Autodesk Inventor part; units mm, degrees
ref_plane "YZ Plane" through (0, 0, 0) normal (1, 0, 0) x (0, 1, 0)
ref_plane "XZ Plane" through (0, 0, 0) normal (0, 1, 0) x (-1, 0, 0)
ref_plane "XY Plane" through (0, 0, 0) normal (0, 0, 1) x (1, 0, 0)
sketch "Sketch1" plane through (0, 0, 0) normal (1, 0, 0) x (0, 1, 0)
  circle A0 centre (0, 0) radius 2.5
extrude "Extrusion1" add sketch "Sketch1" along normal mid plane 3
sketch "Sketch2" plane through (1.5, 0, 0) normal (1, 0, 0) x (0, 0, -1)
  circle A0 centre (0, 0) radius 1.5
extrude "Extrusion2" add sketch "Sketch2" along normal blind 18
fillet "Fillet1" radius 1.2 1 edges at (-1.5, -2.5, 0)
sketch "Sketch3" plane through (0, 0, 0) normal (0, 1, 0) x (-1, 0, 0)
  line L0 (1.5, 1.3) -> (1.5, -1.3)
  line L1 (0.3, -2.5) -> (0.3, 2.5)
  line L2 (1.5, 0.5) -> (0.3, 0.5)
  line L3 (1.5, -0.5) -> (0.3, -0.5)
  line L4 (1.5, -0.5) -> (1.5, 0.5)
  line L5 (0.3, 0.5) -> (0.3, -0.5)
  point P0 (0, 0)
extrude "Extrusion3" cut sketch "Sketch3" along normal mid plane 18
thread "Thread1"
thread "Thread2"
properties part number "parafuso do captador( necessita de reparo)"
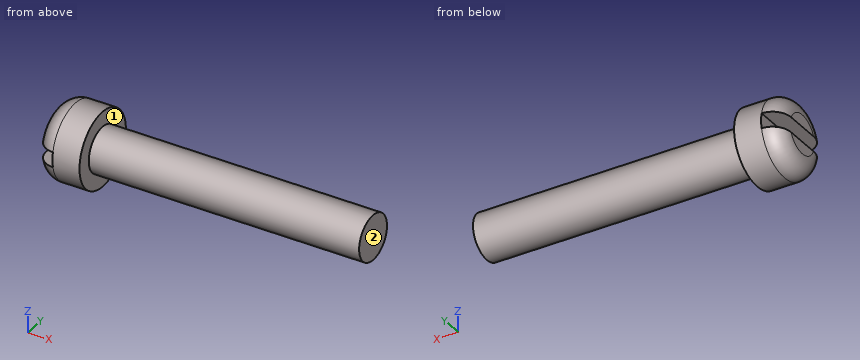
Work out the finished part from the listing and answer in its coordinate system (mm). Face numbers are marked on the shaded views. A direction names the side the tool comes from. Round coordinates to 2 decimals unless told otherwise and drop trailing zeros. Loops run counter-clockwise (first coordinate to the right, second up) from the corner with the lowest first, then second, coordinate; pieces in that order, holes last. Notation, with made-up numbers: M -20,-23.75 L 26,-23.75 A8 cw 26,-14.75 Z; hole C 44.5,68 d5. An arc over 180 degrees is marked long. One line per question, with ' | ' between items.
Q1. Find section B-B, the plane y = 0. Give the vertices of the cut face in (x, z).
Conclusion:
outline: M -1.5,-1.3 A1.2 ccw -0.3,-2.5 L 1.5,-2.5 L 1.5,-1.5 L 19.5,-1.5 L 19.5,1.5 L 1.5,1.5 L 1.5,2.5 L -0.3,2.5 A1.2 ccw -1.5,1.3 L -1.5,0.5 L -0.3,0.5 L -0.3,-0.5 L -1.5,-0.5 Z
Q2. Find section A-A, the plane z = 0. Give the vertices of the cut face in (x, y).
Conclusion:
outline: M -0.3,-2.5 L 1.5,-2.5 L 1.5,-1.5 L 19.5,-1.5 L 19.5,1.5 L 1.5,1.5 L 1.5,2.5 L -0.3,2.5 Z
Q3. Each of these flat-tipped pins is pushed along its axis until it touches: pin 1 Ø1 at (x, y) = (4.5, -0.5) entering from -Z; pin 2 Ø1.5 at (x, z) = (2, -1.5) entering from -Y; pin 3 Ø3 at (x, z) = (17, -2) entering from -Y. Where does it stop, or does it pass through?
Conclusion:
pin 1: stops at z = -1.5 | pin 2: stops at y = -2.32 | pin 3: stops at y = -1.41
Q4. Find section C-C, the plane x = 15.5. Give the vertices of the cut face in (y, z), then the cut area to 3 significant figures.
Conclusion:
outline: C 0,0 d3 | area: 7.07 mm2
Q5. A tool of negligible diameter and unlimited length cuts with its end or side. For the marked faces 1 and 2, from which of +Z, -Z, +X, -X, +Y, -Y can it reach the whole face along a straight path? Write none if from no direction.
Conclusion:
face 1: +X | face 2: +Z, -Z, +X, +Y, -Y
Q6. Consider line 1 along X through (y, z) = (-0.4, 0.45); line 2 along X through (y, z) = (1.9, 0); line 3 along Y through (x, z) = (12, -0.1). Determine where each line is inside the solid, lowest interval first. Write a range as from..to.
Conclusion:
line 1: x = -0.3..19.5 | line 2: x = -0.3..1.5 | line 3: y = -1.5..1.5
